```python
from build123d import *

# Parameters (mm, degrees)
SKETCH8_W                           = 120
SKETCH8_H                           = 150
BOSS_EXTRUDE3_DEPTH                 = 5
SKETCH9_R                           = 50
BOSS_EXTRUDE4_DEPTH                 = 5
BOSS_EXTRUDE8_DEPTH                 = 3
BOSS_EXTRUDE8_DEPTH_BACK            = 0.0001
SKETCH29_R                          = 3
CUT_EXTRUDE9_OUTLINE_R              = 3
CUT_EXTRUDE9_DEPTH                  = 0.01
F_7_32_0_21875_DIAMETER_HOLE1_D     = 3.2
F_7_32_0_21875_DIAMETER_HOLE1_DEPTH = 5
F_7_32_0_21875_DIAMETER_HOLE1_TIP   = 0.96137699
FILLET3_R                           = 4
SKETCH38_W                          = 26
SKETCH38_H                          = 70
CUT_EXTRUDE10_DEPTH                 = 40
SKETCH39_W                          = 25
SKETCH39_H                          = 18
CUT_EXTRUDE11_DEPTH                 = 40


# Read off the part's stored shape, not the designer's step: Cut-Extrude9
with BuildPart() as part:
    # Sketch8 → Boss-Extrude3 (new body)
    with BuildSketch(Plane(origin=(0, 0, 0), x_dir=(1, 0, 0), z_dir=(0, 1, 0))):
        with Locations((73.708855083, 72.164227744)):
            Rectangle(SKETCH8_W, SKETCH8_H)
    extrude(amount=BOSS_EXTRUDE3_DEPTH)

    # Sketch9 → Boss-Extrude4 (add)
    with BuildSketch(Plane(origin=(0, 0, 0), x_dir=(1, 0, 0), z_dir=(0, 1, 0))):
        with Locations((-22.779007595, 70.886233868)):
            Circle(SKETCH9_R)
    extrude(amount=BOSS_EXTRUDE4_DEPTH)

    # Sketch29 → Boss-Extrude8 (add, two sides: drawn at the far end of the back side and taken through both)
    with BuildSketch(Plane(origin=(0, 0, 0), x_dir=(1, 0, 0), z_dir=(0, 1, 0)).offset(-BOSS_EXTRUDE8_DEPTH_BACK)):
        with Locations(Location((19.708855083, 3.164227744, 0), (0, 0, 270))):
            Circle(SKETCH29_R)
    extrude(amount=BOSS_EXTRUDE8_DEPTH + BOSS_EXTRUDE8_DEPTH_BACK)

    # Cut-Extrude9 outline → Cut-Extrude9 (cut)
    with BuildSketch(Plane(origin=(0, 0, 0), x_dir=(1, 0, 0), z_dir=(0, 1, 0))):
        with Locations((127.708855083, 141.164227744)):
            Circle(CUT_EXTRUDE9_OUTLINE_R)
    extrude(amount=CUT_EXTRUDE9_DEPTH, mode=Mode.SUBTRACT)

    # 7/32 (0.21875) Diameter Hole1
    with Locations(Plane(origin=(0, 5, 0), x_dir=(1, 0, 0), z_dir=(0, 1, 0))):
        with Locations((18.917123201, 141.531370062), (127.969984407, 141.269223761), (127.602547564, 3.45328248), (19.774147178, 3.570575466), (-67.115618064, 71.668740496)):
            Hole(F_7_32_0_21875_DIAMETER_HOLE1_D / 2, depth=F_7_32_0_21875_DIAMETER_HOLE1_DEPTH)
            with Locations((0, 0, -(F_7_32_0_21875_DIAMETER_HOLE1_DEPTH + F_7_32_0_21875_DIAMETER_HOLE1_TIP / 2))):  # 118° drill point
                Cone(0, F_7_32_0_21875_DIAMETER_HOLE1_D / 2, F_7_32_0_21875_DIAMETER_HOLE1_TIP, mode=Mode.SUBTRACT)

    # Fillet3
    fillet3_edges = [part.edges().sort_by_distance(p)[0] for p in [
        (13.708855083, 2.5, -147.164227744),
        (133.708855083, 2.5, -147.164227744),
        (133.708855083, 2.5, 2.835772256),
        (13.708855083, 2.5, 2.835772256),
    ]]
    fillet(fillet3_edges, radius=FILLET3_R)

    # Sketch38 → Cut-Extrude10 (cut)
    with BuildSketch(Plane(origin=(0, 5, 0), x_dir=(1, 0, 0), z_dir=(0, 1, 0))):
        with Locations((-21.291144917, 72.164227744)):
            Rectangle(SKETCH38_W, SKETCH38_H)
    extrude(amount=-CUT_EXTRUDE10_DEPTH, mode=Mode.SUBTRACT)

    # Sketch39 → Cut-Extrude11 (cut)
    with BuildSketch(Plane(origin=(0, 5, 0), x_dir=(1, 0, 0), z_dir=(0, 1, 0))):
        with Locations((44.875898376, 128.991672485)):
            Rectangle(SKETCH39_W, SKETCH39_H)
    extrude(amount=-CUT_EXTRUDE11_DEPTH, mode=Mode.SUBTRACT)


solid = part.part
```
Model file for the job. Use its own axes, mm. A direction names the side the tool comes from. Give positions to 0.01 mm unless a question says otherwise; leave off trailing zeros. Write each loop counter-clockwise with the first axis right and the second up, starting at its lowest first coordinate (ties: lowest second). Pieces come first, ordered by that corner, then holes. Notation, with made-up numbers: (36, 35.25) - (43, 35.25) arc R22 ccw to (43, 51.25) - close; hole circle Ø11 at (25.25, -5.75). An arc over 180 degrees is marked (long way). One line per question, with ' | ' between items. Start each with the question number.
(1) Slice it at A-A on z = -129. Write the cut outline in (x, y).
(2) Wall check: line 1 along X through (y, z) = (2.2, -127); line 2 along X through (y, z) = (2.25, -12); line 3 along X through (y, z) = (0.5, -53.5). Give the ranges that are in metal, low to high. Write a range as from..to.
(3) Slice it at B-B on x = 49. Write the cut outline in (y, z).
(4) 3-axis set-ups, long thin cutter, end or side, ignore diameter. For faces 4 (the face through (45, 3, -119.992)), 5 (the face through (13.709, 2, -124)), 6 (the face through (13.709, 2, -19)): which of +Z, -Z, +X, -X, +Y, -Y reach the whole face in a straight line?
(5) Pin check, flat tips, straight feed: P1, Ø10, axis at x = 36, z = -41.5, coming from the -Y side; P2, Ø1, axis at x = -51.5, y = 1, coming from the -Z side; P3, Ø1.5, axis at y = 2.5, z = -68.5, coming from the -X side; P4, Ø1.5, axis at y = 1, z = -41, coming from the -X side. Stop position of each tip, or through.
(6) Slice it at C-C on y = 0.8. Write the cut outline in (x, z).
(7) Two-plate mould, pull along Z, no slides. Class faces 1 (the face through (14.85, 2.54, -145.96)), 2 (the face through (-21, 3, -37.164)), 3 (the face through (133.709, 2, -71)): +Z half, -Z half, draft (parallel to the pull), parting line (faces both ways), or undercut.
Results below:
1) outline: (13.71, 0) - (32.38, 0) - (32.38, 5) - (13.71, 5) - close; (57.38, 0) - (133.71, 0) - (133.71, 5) - (57.38, 5) - close
2) line 1: 13.71..32.38, 57.38..133.71 | line 2: 13.71..133.71 | line 3: -69.66..-34.29, -8.29..133.71
3) outline: (0, -147.16) - (5, -147.16) - (5, -137.99) - (0, -137.99) - close; (0, -119.99) - (5, -119.99) - (5, 2.84) - (0, 2.84) - close
4) face 4: +Y, -Y | face 5: -Z, +Y, -Y | face 6: +Z, +Y, -Y
5) P1: y = 0 | P2: z = -112.16 | P3: x = -72.75 | P4: x = -63.41
6) outline: (13.71, -143.16) arc R4 ccw to (17.71, -147.16) - (129.71, -147.16) arc R4 ccw to (133.71, -143.16) - (133.71, -1.16) arc R4 ccw to (129.71, 2.84) - (17.71, 2.84) arc R4 ccw to (13.71, -1.16) - (13.71, -36.7) arc R50 ccw (long way) to (13.71, -105.07) - close; hole circle Ø3.2 at (-67.12, -71.67); hole (-34.29, -107.16) - (-8.29, -107.16) - (-8.29, -37.16) - (-34.29, -37.16) - close; hole circle Ø3.2 at (18.92, -141.53); hole circle Ø3.2 at (19.77, -3.57); hole (32.38, -137.99) - (57.38, -137.99) - (57.38, -119.99) - (32.38, -119.99) - close; hole circle Ø3.2 at (127.6, -3.45); hole circle Ø3.2 at (127.97, -141.27)
7) face 1: -Z half | face 2: undercut | face 3: draft
